Verification items for the finished model (mm, model axes). A direction names the side the tool comes from. Coordinates: 2 decimals unless noted, no trailing zeros.
Q1. Cross-section at A-A, the plane y = 0. Count the separate pieces of the cut face and the enclosed holes in it, and give its area (3 significant figures).
Q2. Thickness scan on line 1 (Y direction, x = 0, z = 9.75); line 2 (Y direction, x = -2.5, z = 9.5); line 3 (X direction, y = -22, z = 2). Record the ranges inside material, lowest first.
Q3. Set-up check for faces 1 (the flat face through (45.07, 35.06, 10.99)), 2 (the cylindrical face through (-53.245, 0.231, 11.014)), 3 (the cylindrical face through (-22.897, -46.056, 4.388)), 4 (the conical face through (-24.89, 25.06, 1.43)), 5 (the flat face through (25, 42, 6)): record each of +Z, -Z, +X, -X, +Y, -Y from which the full face is reachable in a straight line by a thin tool's end or side.
Q4. Depth check by flat-ended pin: P1, Ø13.5, axis at x = -43.5, y = -20.29, coming from the -Z side; P2, Ø3, axis at x = -45.5, y = -18.5, coming from the +Z side; P3, Ø8, axis at y = 29, z = 6.5, coming from the -X side; P4, Ø8, axis at x = -14, y = -21.5, coming from the -Z side. Enter the tip coordinate at first touch or a pass-through.
Q5. Draft check along X on faces 6 (the cylindrical face through (-56, 0, 5)), 7 (the cylindrical face through (46.05, 20.17, 5.07)), 8 (the cylindrical face through (56, 0, 5)). Enter one of: pulls with the +X half, pulls with the -X half, needs draft (parallel to the pull), parting line crosses it, or undercut.
from build123d import *

# Parameters (mm, degrees)
EXTRUDE_1_DEPTH     = 12
SKETCH_3_R          = 2.65
CUT_EXTRUDE_1_DEPTH = 8
SKETCH_5_R          = 2.55
SKETCH_5_R_2        = 3.1
CUT_EXTRUDE_2_DEPTH = 77.026311235
SKETCH_7_R          = 5.25
CUT_EXTRUDE_3_DEPTH = 2
CHAMFER_3_SIZE      = 2
CUT_EXTRUDE_4_DEPTH = 12
SKETCH_9_R          = 39.85
SKETCH_9_R_2        = 36.85
EXTRUDE_2_DEPTH     = 4
SKETCH_10_R         = 2
CUT_EXTRUDE_5_DEPTH = 8
CHAMFER_4_SIZE      = 2
CHAMFER_5_SIZE      = 0.5


with BuildPart() as part:
    # Эскиз2 → Бобышка-Вытянуть1 (new body)
    with BuildSketch(Plane.XY):
        with BuildLine():
            Line((40, 50), (-40, 50))
            Line((-40, 50), (-51.798872756, 21.280901795))
            ThreePointArc((-51.798872756, 21.280901795), (-56, 0), (-51.798872756, -21.280901795))
            Line((-51.798872756, -21.280901795), (-40, -50))
            Line((-40, -50), (40, -50))
            Line((40, -50), (51.798872756, -21.280901795))
            ThreePointArc((51.798872756, -21.280901795), (56, 0), (51.798872756, 21.280901795))
            Line((51.798872756, 21.280901795), (40, 50))
        make_face()
    extrude(amount=EXTRUDE_1_DEPTH)

    # Эскиз3 → Вырез-Вытянуть1 (cut)
    with BuildSketch(Plane(origin=(0, 50, 0), x_dir=(1, 0, 0), z_dir=(0, 1, 0))):
        with Locations(Location((-25, -6, 0), (0, 0, 180))):
            Circle(SKETCH_3_R)
        with Locations(Location((0, -6, 0), (0, 0, 180))):
            Circle(SKETCH_3_R)
        with Locations(Location((25, -6, 0), (0, 0, 180))):
            Circle(SKETCH_3_R)
    cut_extrude_1 = extrude(amount=-CUT_EXTRUDE_1_DEPTH, mode=Mode.SUBTRACT)

    # Зеркальное отражение1: Вырез-Вытянуть1 across plane
    add(cut_extrude_1.mirror(Plane.ZX), mode=Mode.SUBTRACT)

    # Эскиз5 → Вырез-Вытянуть2 (cut, through all)
    with BuildSketch(Plane.XY.offset(12)):
        with Locations((-48, 0)):
            Circle(SKETCH_5_R)
        with Locations((-43.502773778, 20.285676564)):
            Circle(SKETCH_5_R)
        with Locations((-43.502773778, -20.285676564)):
            Circle(SKETCH_5_R)
        with Locations((-30.853805265, -36.77013327)):
            Circle(SKETCH_5_R_2)
        with Locations((-30.853805265, 36.77013327)):
            Circle(SKETCH_5_R_2)
        with Locations(Location((30.853805265, 36.77013327, 0), (0, 0, 180))):
            Circle(SKETCH_5_R_2)
        with Locations(Location((30.853805265, -36.77013327, 0), (0, 0, 180))):
            Circle(SKETCH_5_R_2)
        with Locations(Location((43.502773778, -20.285676564, 0), (0, 0, 180))):
            Circle(SKETCH_5_R)
        with Locations(Location((43.502773778, 20.285676564, 0), (0, 0, 180))):
            Circle(SKETCH_5_R)
        with Locations(Location((48, 0, 0), (0, 0, 180))):
            Circle(SKETCH_5_R)
    extrude(amount=-CUT_EXTRUDE_2_DEPTH, mode=Mode.SUBTRACT)

    # Эскиз7 → Вырез-Вытянуть3 (cut)
    with BuildSketch(Plane.XY.offset(12)):
        with Locations((-43.502773778, 20.285676564)):
            Circle(SKETCH_7_R)
        with Locations((-48, 0)):
            Circle(SKETCH_7_R)
        with Locations((-43.502773778, -20.285676564)):
            Circle(SKETCH_7_R)
        with Locations((43.502773778, 20.285676564)):
            Circle(SKETCH_7_R)
        with Locations((48, 0)):
            Circle(SKETCH_7_R)
        with Locations((43.502773778, -20.285676564)):
            Circle(SKETCH_7_R)
    extrude(amount=-CUT_EXTRUDE_3_DEPTH, mode=Mode.SUBTRACT)

    # Фаска3
    chamfer_3_edges = [part.edges().sort_by_distance(p)[0] for p in [
        (0, -50, 12),
        (45.899436378, -35.640450898, 12),
        (56, 0, 12),
        (45.899436378, 35.640450898, 12),
        (0, 50, 12),
        (-45.899436378, 35.640450898, 12),
        (-56, 0, 12),
        (-45.899436378, -35.640450898, 12),
    ]]
    chamfer(chamfer_3_edges, length=CHAMFER_3_SIZE)

    # Эскиз8 → Вырез-Вытянуть4 (cut)
    with BuildSketch(Plane.XY.offset(12)):
        with BuildLine():
            Line((-17.5, -27.5), (17.5, -27.5))
            ThreePointArc((17.5, -27.5), (24.571067812, -24.571067812), (27.5, -17.5))
            Line((27.5, -17.5), (27.5, 17.5))
            ThreePointArc((27.5, 17.5), (24.571067812, 24.571067812), (17.5, 27.5))
            Line((17.5, 27.5), (-17.5, 27.5))
            ThreePointArc((-17.5, 27.5), (-24.571067812, 24.571067812), (-27.5, 17.5))
            Line((-27.5, 17.5), (-27.5, -17.5))
            ThreePointArc((-27.5, -17.5), (-24.571067812, -24.571067812), (-17.5, -27.5))
        make_face()
    extrude(amount=-CUT_EXTRUDE_4_DEPTH, mode=Mode.SUBTRACT)

    # Эскиз9 → Бобышка-Вытянуть2 (add)
    with BuildSketch(Plane(origin=(0, 0, 0), x_dir=(-1, 0, 0), z_dir=(0, 0, -1))):
        Circle(SKETCH_9_R)
        Circle(SKETCH_9_R_2, mode=Mode.SUBTRACT)
    extrude(amount=EXTRUDE_2_DEPTH)

    # Эскиз10 → Вырез-Вытянуть5 (cut)
    with BuildSketch(Plane.XY.offset(12)):
        with Locations((0, 32.5)):
            Circle(SKETCH_10_R)
        with Locations((32.5, 0)):
            Circle(SKETCH_10_R)
        with Locations((0, -32.5)):
            Circle(SKETCH_10_R)
        with Locations((-32.5, 0)):
            Circle(SKETCH_10_R)
    extrude(amount=-CUT_EXTRUDE_5_DEPTH, mode=Mode.SUBTRACT)

    # Фаска4
    chamfer_4_edges = [part.edges().sort_by_distance(p)[0] for p in [
        (24.571067812, 24.571067812, 0),
        (27.5, 0, 0),
        (24.571067812, -24.571067812, 0),
        (0, -27.5, 0),
        (-24.571067812, -24.571067812, 0),
        (-27.5, 0, 0),
        (-24.571067812, 24.571067812, 0),
        (0, 27.5, 0),
    ]]
    chamfer(chamfer_4_edges, length=CHAMFER_4_SIZE)

    # Фаска5
    chamfer_5_edges = [part.edges().sort_by_distance(p)[0] for p in [
        (39.85, 0, -4),
    ]]
    chamfer(chamfer_5_edges, length=CHAMFER_5_SIZE)


solid = part.part
Check values:
1. separate pieces: 4
1. enclosed holes: 0
1. area: 492 mm2
2. line 1: y = -50 to -34.5, -30.5 to -27.5, 27.5 to 30.5, 34.5 to 50
2. line 2: y = -50 to -27.5, 27.5 to 50
2. line 3: x = -51.5 to -45.39, -41.62 to -26.43, 26.43 to 41.62, 45.39 to 51.5
3. face 1: +Z, +X, +Y
3. face 2: +Z
3. face 3: -Y
3. face 4: -Z
3. face 5: +Y
4. P1: stops at z = 0
4. P2: stops at z = 10
4. P3: stops at x = -50.27
4. P4: passes through
5. face 6: pulls with the -X half
5. face 7: undercut
5. face 8: pulls with the +X half
